Read the model definition and answer for the solid it produces. Units are mm, in the model's axes. A direction names the side the tool comes from. Coordinates: 2 decimals unless noted, no trailing zeros. Loops run counter-clockwise (first coordinate to the right, second up) from the corner with the lowest first, then second, coordinate; pieces in that order, holes last. Notation, with made-up numbers: (-30, 68) -> (25, 68) arc R9 cw to (25, 81) -> close; hole circle Ø11 at (-28, 83.25). An arc over 180 degrees is marked (long way). Answer as a JSON object with one key per item and string values. Group by question number.
Q1. For faces 1 (the flat face through (26, 19, -2)), 2 (the flat face through (-26, 19, -2)), 3 (the flat face through (0, 16, -21)), 4 (the flat face through (0, 17, 1)), 5 (the flat face through (-1, 6, -27)), determine the directions among +Z, -Z, +X, -X, +Y, -Y from which every point of the face is accessible in a straight line to the end or side of a thin tool.
Q2. The part is cut by section A-A on z = -17. Write down the section's boundary in (x, y), and give its area (3 significant figures).
Q3. The part is cut by section D-D on y = 26. Write down the section's boundary in (x, z), and give its area (3 significant figures).
Q4. Straight lines are drawn through the part: line 1 along Z through (x, y) = (44, 2.5); line 2 along X through (y, z) = (4.5, -17); line 3 along Y through (x, z) = (4, 7). For each, find the intervals that lie inside material, in ascending order. Write a range as [from, to].
Q5. Determine the mould class of faces 6 (the flat face through (-21, 28, -13.212)), 7 (the cylindrical face through (-40.034, 5.577, -17.521)), 8 (the cylindrical face through (-40.034, 5.577, 7.479)), 9 (the flat face through (-1, 6, 27)) for opening direction Z: released by +Z, released by -Z, zero draft, split by the parting line, or undercut.
Q6. The part is cut by section B-B on y = 2. Write down the section's boundary in (x, z).
Q7. Each of these flat-tipped pins is pushed along its axis until it touches: P1, Ø20, axis at x = 4, z = 5.5, coming from the +Y side (3 decimals); P2, Ø10.5, axis at y = 23.5, z = 11, coming from the -X side; P3, Ø2.5, axis at x = -19.5, z = -18.5, coming from the +Y side; P4, Ø6.5, axis at x = -44, z = -17, coming from the +Y side. Where does it stop, or does it pass through?
Q8. The part is cut by section C-C on x = 21.5. Write down the section's boundary in (y, z), and give its area (3 significant figures).
from build123d import *

# Parameters (mm, degrees)
BOSS_EXTRUDE1_DEPTH = 27
CUT_EXTRUDE1_DEPTH  = 116.83177457
SKETCH3_R           = 4
CUT_EXTRUDE2_DEPTH  = 64.921827258
FILLET1_R           = 10


with BuildPart() as part:
    # Sketch1 → Boss-Extrude1 (new, symmetric)
    with BuildSketch(Plane.XY):
        Polygon((-54, 0), (0, 0), (0, 11), (-26, 11), (-54, 11), align=None)
        Polygon((-26, 11), (0, 11), (0, 17), (-9, 17), (-13.235294044, 24.941176333), (-17, 32), (-26, 32), align=None)
        Polygon((0, 11), (0, 0), (54, 0), (54, 11), (26, 11), align=None)
        Polygon((0, 17), (0, 11), (26, 11), (26, 32), (17, 32), (13.235294044, 24.941176333), (9, 17), align=None)
    extrude(amount=BOSS_EXTRUDE1_DEPTH, both=True)

    # Sketch2 → Cut-Extrude1 (cut, through all)
    with BuildSketch(Plane(origin=(54, 0, 0), x_dir=(0, 0, -1), z_dir=(1, 0, 0))):
        with BuildLine():
            Line((-27, 32), (-27, 11))
            ThreePointArc((-27, 11), (-9.470653919, 26.433857761), (13.211938526, 32))
            Line((13.211938526, 32), (-27, 32))
        make_face()
        Polygon((21, 23), (21, 11), (27, 11), (27, 32), (13.211938526, 32), (13.211938526, 23), align=None)
    extrude(amount=-CUT_EXTRUDE1_DEPTH, mode=Mode.SUBTRACT)

    # Sketch3 → Cut-Extrude2 (cut, through all)
    with BuildSketch(Plane(origin=(0, 11, 0), x_dir=(1, 0, 0), z_dir=(0, 1, 0))):
        with Locations(Location((-44, 17, 0), (0, 0, 270))):
            Circle(SKETCH3_R)
        with Locations(Location((-44, -8, 0), (0, 0, 270))):
            Circle(SKETCH3_R)
        with Locations(Location((44, -8, 0), (0, 0, 90))):
            Circle(SKETCH3_R)
        with Locations(Location((44, 17, 0), (0, 0, 90))):
            Circle(SKETCH3_R)
    extrude(amount=-CUT_EXTRUDE2_DEPTH, mode=Mode.SUBTRACT)

    # Fillet1
    fillet1_edges = [part.edges().sort_by_distance(p)[0] for p in [
        (-54, 5.5, 27),
        (54, 5.5, 27),
    ]]
    fillet(fillet1_edges, radius=FILLET1_R)


solid = part.part
Final values:
{
 "1": {"face 1": "+Z, -Z, +X, +Y", "face 2": "+Z, -Z, -X, +Y", "face 3": "-Z, +X, -X, +Y", "face 4": "+Z, -Z, +Y", "face 5": "-Z, +X, -X, +Y, -Y"},
 "2": {"outline": "(-54, 0) -> (-48, 0) -> (-48, 11) -> (-54, 11) -> close; (-40, 0) -> (40, 0) -> (40, 11) -> (26, 11) -> (26, 23) -> (12.2, 23) -> (9, 17) -> (-9, 17) -> (-12.2, 23) -> (-26, 23) -> (-26, 11) -> (-40, 11) -> close; (48, 0) -> (54, 0) -> (54, 11) -> (48, 11) -> close", "area": "1,510 mm2"},
 "3": {"outline": "(-26, -13.21) -> (-13.8, -13.21) -> (-13.8, 10.28) -> (-26, 10.28) -> close; (13.8, -13.21) -> (26, -13.21) -> (26, 10.28) -> (13.8, 10.28) -> close", "area": "573 mm2"},
 "4": {"line 1": "z = [-27, -21], [-13, 4], [12, 27]", "line 2": "x = [-54, -48], [-40, 40], [48, 54]", "line 3": "y = [0, 17]"},
 "5": {"face 6": "released by -Z", "face 7": "undercut", "face 8": "undercut", "face 9": "released by +Z"},
 "6": {"outline": "(-54, -27) -> (54, -27) -> (54, 17) arc R10 ccw to (44, 27) -> (-44, 27) arc R10 ccw to (-54, 17) -> close; hole circle Ø8 at (-44, -17); hole circle Ø8 at (-44, 8); hole circle Ø8 at (44, -17); hole circle Ø8 at (44, 8)"},
 "7": {"P1": "stops at y = 26.375", "P2": "stops at x = -26", "P3": "stops at y = 23", "P4": "passes through"},
 "8": {"outline": "(0, -27) -> (11, -27) -> (11, -21) -> (23, -21) -> (23, -13.21) -> (32, -13.21) arc R49 ccw to (11, 27) -> (0, 27) -> close", "area": "1,280 mm2"}
}
